Work out the finished part from the listing and answer in its coordinate system (mm). Round coordinates to 2 decimals unless told otherwise and drop trailing zeros. Write each loop counter-clockwise with the first axis right and the second up, starting at its lowest first coordinate (ties: lowest second). Pieces come first, ordered by that corner, then holes. Notation, with made-up numbers: M 13.25,-18.75 L 33.25,-18.75 A34 ccw 33.25,14.25 Z; hole C 32.25,-15.75 d5. An arc over 180 degrees is marked long. One line per item, written item: value. Start each with the question number.
Q1. Find section C-C (x = -160). Write down the section's boundary in (y, z).
Q2. Find section B-B (y = 0). Count the separate pieces of the cut face and the enclosed holes in it, and give its area (3 significant figures).
Q3. Given pin 1 Ø5.5 at (x, z) = (-254, 129.54) entering from +Y; pin 2 Ø1 at (x, y) = (-173.5, -0.5) entering from -Z, each flat-ended and moving along its own axis, determine where each tip first touches the part or whether it passes through.
Q4. Consider probe 1 along X at (y, z) = (0.55, 18.5); probe 2 along X at (y, z) = (-0.2, 129.54); probe 3 along Z at (x, y) = (254, 0.45). Determine where each line is inside the solid, lowest interval first.
Q5. Find section A-A (z = 92). Write down the section's boundary in (x, y).
from build123d import *

# Parameters (mm, degrees)
SKETCH1_W           = 546.1
SKETCH1_H           = 3.175
BOSS_EXTRUDE1_DEPTH = 184.15
SKETCH2_R           = 2.413
CUT_EXTRUDE2_DEPTH  = 4.175
SKETCH5_W           = 546.1
SKETCH5_H           = 3.175
BOSS_EXTRUDE2_DEPTH = 12.7
SKETCH6_W           = 76.2
SKETCH6_H           = 127
CUT_EXTRUDE4_DEPTH  = 4.175
SKETCH7_R           = 2.413
CUT_EXTRUDE5_DEPTH  = 4.175


with BuildPart() as part:
    # Sketch1 → Boss-Extrude1 (new body)
    with BuildSketch(Plane.XY):
        Rectangle(SKETCH1_W, SKETCH1_H)
    extrude(amount=BOSS_EXTRUDE1_DEPTH)

    # Sketch2 → Cut-Extrude2 (cut, through all)
    with BuildSketch(Plane(origin=(0, 1.5875, 0), x_dir=(1, 0, 0), z_dir=(0, 1, 0))):
        with Locations((-234.95, -129.54)):
            Circle(SKETCH2_R)
        with Locations((-254, -129.54)):
            Circle(SKETCH2_R)
        with Locations((-254, -7.62)):
            Circle(SKETCH2_R)
        with Locations((-234.95, -7.62)):
            Circle(SKETCH2_R)
        with Locations((254, -7.62)):
            Circle(SKETCH2_R)
        with Locations((234.95, -7.62)):
            Circle(SKETCH2_R)
        with Locations((254, -129.54)):
            Circle(SKETCH2_R)
        with Locations((234.95, -129.54)):
            Circle(SKETCH2_R)
    extrude(amount=-CUT_EXTRUDE2_DEPTH, mode=Mode.SUBTRACT)

    # Sketch5 → Boss-Extrude2 (add)
    with BuildSketch(Plane(origin=(0, 0, 0), x_dir=(-1, 0, 0), z_dir=(0, 0, -1))):
        Rectangle(SKETCH5_W, SKETCH5_H)
    extrude(amount=BOSS_EXTRUDE2_DEPTH)

    # Sketch6 → Cut-Extrude4 (cut, through all)
    with BuildSketch(Plane(origin=(0, 1.5875, 0), x_dir=(1, 0, 0), z_dir=(0, 1, 0))):
        with Locations((-165.1, -50.8)):
            Rectangle(SKETCH6_W, SKETCH6_H)
        with Locations((165.1, -50.8)):
            Rectangle(SKETCH6_W, SKETCH6_H)
    extrude(amount=-CUT_EXTRUDE4_DEPTH, mode=Mode.SUBTRACT)

    # Sketch7 → Cut-Extrude5 (cut, through all)
    with BuildSketch(Plane(origin=(0, 1.5875, 0), x_dir=(1, 0, 0), z_dir=(0, 1, 0))):
        with Locations((-254, -142.24)):
            Circle(SKETCH7_R)
        with Locations((-234.95, -142.24)):
            Circle(SKETCH7_R)
        with Locations((254, -142.24)):
            Circle(SKETCH7_R)
        with Locations((234.95, -142.24)):
            Circle(SKETCH7_R)
    extrude(amount=-CUT_EXTRUDE5_DEPTH, mode=Mode.SUBTRACT)


solid = part.part
The answers:
1. outline: M -1.59,114.3 L 1.59,114.3 L 1.59,184.15 L -1.59,184.15 Z
2. separate pieces: 1
2. enclosed holes: 12
2. area: 87,900 mm2
3. pin 1: y = 1.59
3. pin 2: z = 114.3
4. probe 1: -273.05 to -203.2, -127 to 127, 203.2 to 273.05
4. probe 2: -273.05 to -256.41, -251.59 to -237.36, -232.54 to 232.54, 237.36 to 251.59, 256.41 to 273.05
4. probe 3: -12.7 to 5.21, 10.03 to 127.13, 131.95 to 139.83, 144.65 to 184.15
5. outline: M -273.05,-1.59 L -203.2,-1.59 L -203.2,1.59 L -273.05,1.59 Z; M -127,-1.59 L 127,-1.59 L 127,1.59 L -127,1.59 Z; M 203.2,-1.59 L 273.05,-1.59 L 273.05,1.59 L 203.2,1.59 Z
